from build123d import *

# Parameters (mm, degrees)
BOSS_EXTRUDE4_DEPTH = 5
SKETCH6_W           = 70
SKETCH6_H           = 70
BOSS_EXTRUDE5_DEPTH = 30
SKETCH8_R           = 3
CUT_EXTRUDE1_DEPTH  = 2
CUT_EXTRUDE2_START  = -30
CUT_EXTRUDE2_DEPTH  = 30
SKETCH10_W          = 140
SKETCH10_H          = 70
BOSS_EXTRUDE6_DEPTH = 2.5
FILLET1_R           = 10
CHAMFER1_SIZE       = 1.25
CHAMFER2_SIZE       = 1.25


with BuildPart() as part:
    # Sketch5 → Boss-Extrude4 (new body)
    with BuildSketch(Plane(origin=(0, 0, 0), x_dir=(1, 0, 0), z_dir=(0, 1, 0))):
        with BuildLine():
            Line((-22.5, -32.5), (22.5, -32.5))
            ThreePointArc((22.5, -32.5), (29.571067812, -29.571067812), (32.5, -22.5))
            Line((32.5, -22.5), (32.5, 22.5))
            ThreePointArc((32.5, 22.5), (29.571067812, 29.571067812), (22.5, 32.5))
            Line((22.5, 32.5), (-22.5, 32.5))
            ThreePointArc((-22.5, 32.5), (-29.571067812, 29.571067812), (-32.5, 22.5))
            Line((-32.5, 22.5), (-32.5, -22.5))
            ThreePointArc((-32.5, -22.5), (-29.571067812, -29.571067812), (-22.5, -32.5))
        make_face()
    extrude(amount=BOSS_EXTRUDE4_DEPTH)

    # Sketch6 → Boss-Extrude5 (add)
    with BuildSketch(Plane(origin=(0, 5, 0), x_dir=(1, 0, 0), z_dir=(0, 1, 0))):
        Rectangle(SKETCH6_W, SKETCH6_H)
    extrude(amount=BOSS_EXTRUDE5_DEPTH)

    # Sketch8 → Cut-Extrude1 (cut)
    with BuildSketch(Plane.XZ):
        with Locations(Location((26.037533906, -26.035533906, 0), (0, 0, 270))):
            Circle(SKETCH8_R)
        with Locations(Location((26.036533906, 26.036533906, 0), (0, 0, 270))):
            Circle(SKETCH8_R)
        with BuildLine():
            ThreePointArc((-23.035533906, 26.035533906), (-24.887483609, 28.807172503), (-28.156854249, 28.156854249))
            Line((-28.156854249, 28.156854249), (-23.914213562, 23.914213562))
            ThreePointArc((-23.914213562, 23.914213562), (-23.263895308, 24.887483609), (-23.035533906, 26.035533906))
        make_face()
        with BuildLine():
            Line((-23.914213562, 23.914213562), (-28.156854249, 28.156854249))
            ThreePointArc((-28.156854249, 28.156854249), (-28.156854249, 23.914213562), (-23.914213562, 23.914213562))
        make_face()
        with Locations(Location((-26.034533906, -26.036533906, 0), (0, 0, 270))):
            Circle(SKETCH8_R)
    extrude(amount=-CUT_EXTRUDE1_DEPTH, mode=Mode.SUBTRACT)

    # Mirror1: part across plane


with BuildPart() as part_1:
    add(part.part)
    add(part.part.mirror(Plane(origin=(-35, 35, -35), x_dir=(0, 0, 1), z_dir=(1, 0, 0))))

    # Sketch9 → Cut-Extrude2 (cut)
    with BuildSketch(Plane(origin=(0, 35, 0), x_dir=(1, 0, 0), z_dir=(0, 1, 0)).offset(CUT_EXTRUDE2_START)):
        with BuildLine():
            Line((22.5, 32.5), (-92.5, 32.5))
            ThreePointArc((-92.5, 32.5), (-99.571067812, 29.571067812), (-102.5, 22.5))
            Line((-102.5, 22.5), (-102.5, -22.5))
            ThreePointArc((-102.5, -22.5), (-99.571067812, -29.571067812), (-92.5, -32.5))
            Line((-92.5, -32.5), (22.5, -32.5))
            ThreePointArc((22.5, -32.5), (29.571067812, -29.571067812), (32.5, -22.5))
            Line((32.5, -22.5), (32.5, 22.5))
            ThreePointArc((32.5, 22.5), (29.571067812, 29.571067812), (22.5, 32.5))
        make_face()
    extrude(amount=CUT_EXTRUDE2_DEPTH, mode=Mode.SUBTRACT)


with BuildPart() as cut_extrude2_piece_1:
    # of the separate pieces the step leaves, piece 1, a body of its own (cut_extrude2_pieces)
    add(part_1.part.solids().sort_by_distance((35, 5, -35))[0])



with BuildPart() as cut_extrude2_piece_2:
    # of the separate pieces the step leaves, piece 2, a body of its own (cut_extrude2_pieces)
    add(part_1.part.solids().sort_by_distance((-22.5, 0, 32.5))[0])


with BuildPart() as cut_extrude2_piece_3:
    # of the separate pieces the step leaves, piece 3, a body of its own (cut_extrude2_pieces)
    add(part_1.part.solids().sort_by_distance((-92.5, 0, -32.5))[0])


with BuildPart() as cut_extrude2_piece_1_1:
    add(cut_extrude2_piece_1.part)

    add(cut_extrude2_piece_2.part)  # Boss-Extrude6 merges Cut-Extrude2 piece 2

    add(cut_extrude2_piece_3.part)  # Boss-Extrude6 merges Cut-Extrude2 piece 3
    # Sketch10 → Boss-Extrude6 (add)
    with BuildSketch(Plane.XZ.offset(-5)):
        with Locations((-35, 0)):
            Rectangle(SKETCH10_W, SKETCH10_H)
    extrude(amount=-BOSS_EXTRUDE6_DEPTH)

    # Fillet1
    fillet1_edges = [cut_extrude2_piece_1_1.edges().sort_by_distance(p)[0] for p in [
        (35, 20, 35),
        (35, 20, -35),
        (-105, 20, 35),
        (-105, 20, -35),
    ]]
    fillet(fillet1_edges, radius=FILLET1_R)

    # Chamfer1
    chamfer1_edges = [cut_extrude2_piece_1_1.edges().sort_by_distance(p)[0] for p in [
        (29.571067812, 7.5, -29.571067812),
        (-35, 7.5, -32.5),
        (-99.571067812, 7.5, -29.571067812),
        (-102.5, 7.5, 0),
        (-99.571067812, 7.5, 29.571067812),
        (-35, 7.5, 32.5),
        (29.571067812, 7.5, 29.571067812),
        (32.5, 7.5, 0),
    ]]
    chamfer(chamfer1_edges, length=CHAMFER1_SIZE)

    # Chamfer2
    chamfer2_edges = [cut_extrude2_piece_1_1.edges().sort_by_distance(p)[0] for p in [
        (-99.571067812, 35, 29.571067812),
        (-35, 35, 32.5),
        (29.571067812, 35, 29.571067812),
        (32.5, 35, 0),
        (29.571067812, 35, -29.571067812),
        (-35, 35, -32.5),
        (-99.571067812, 35, -29.571067812),
        (-102.5, 35, 0),
    ]]
    chamfer(chamfer2_edges, length=CHAMFER2_SIZE)


solid = cut_extrude2_piece_1_1.part
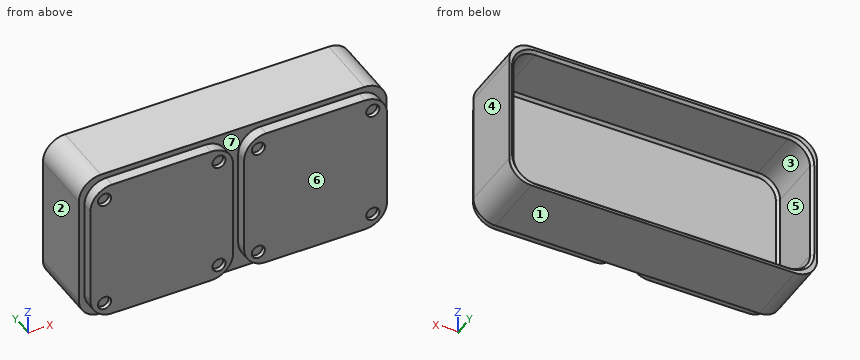
Verification items for the finished model (mm, model axes). Face numbers are marked on the shaded views. A direction names the side the tool comes from. Round coordinates to 2 decimals unless told otherwise and drop trailing zeros. Loops run counter-clockwise (first coordinate to the right, second up) from the corner with the lowest first, then second, coordinate; pieces in that order, holes last. Notation, with made-up numbers: (-6, -27) - (6, -27) arc R18 cw to (6, -2) - close; hole circle Ø8 at (76.25, 8.25). An arc over 180 degrees is marked (long way). Answer in a Markdown table with one row per item. Add a question column.
Q1. Gauge pin test, flat ends, axial feed: pin 1 (5.5 mm diameter, centred on x = -75, y = 3, fed in from +Z); pin 2 (10 mm diameter, centred on x = -65.5, z = 12, fed in from +Y); pin 3 (1.5 mm diameter, centred on y = 1.5, z = -11, fed in from +X); pin 4 (3 mm diameter, centred on x = -44, z = -26.5, fed in from -Y). Record the tip position at first contact, or that the pin passes through.
Q2. Section check A-A on x = -83. Enter the section's corners in (y, z).
Q3. Material ranges on line 1 (X direction, y = 17.5, z = 1.5); line 2 (Z direction, x = 15.5, y = 27.5); line 3 (Y direction, x = 20, z = 22), recorded low to high.
Q4. Tool access check on the marked faces 5, 6 and 7. Record the directions out of +Z, -Z, +X, -X, +Y, -Y that give a thin tool (end or side, any length) a straight path to the whole face; none if there is none.
Q5. Section check C-C on z = -2. Enter the section's corners in (x, y), plus the area to 3 significant figures.
Q6. Release check for a two-part mould opening along X. For the marked faces 1, 2, 3 and 4 record: pulls with the +X half, pulls with the -X half, needs draft (parallel to the pull), parting line crosses it, or undercut.
Q7. Section check B-B on y = 12. Enter the section's corners in (x, z), plus the area to 4 significant figures.
Found:
| question | item | result |
|---|---|---|
| 1 | pin 1 | stops at z = 35 |
| 1 | pin 2 | stops at y = 7.5 |
| 1 | pin 3 | stops at x = 32.5 |
| 1 | pin 4 | stops at y = 2 |
| 2 | outline | (0, -32.5) - (5, -32.5) - (5, -35) - (35, -35) - (35, -33.75) - (33.75, -32.5) - (8.75, -32.5) - (7.5, -31.25) - (7.5, 31.25) - (8.75, 32.5) - (33.75, 32.5) - (35, 33.75) - (35, 35) - (5, 35) - (5, 32.5) - (0, 32.5) - close |
| 3 | line 1 | x = -105 to -102.5, 32.5 to 35 |
| 3 | line 2 | z = -35 to -32.5, 32.5 to 35 |
| 3 | line 3 | y = 0 to 7.5 |
| 4 | face 5 | +Y |
| 4 | face 6 | +Z, -Z, +X, -X, -Y |
| 4 | face 7 | -Y |
| 5 | outline | (-105, 5) - (-102.5, 5) - (-102.5, 0) - (-37.5, 0) - (-37.5, 5) - (-32.5, 5) - (-32.5, 0) - (32.5, 0) - (32.5, 5) - (35, 5) - (35, 35) - (33.75, 35) - (32.5, 33.75) - (32.5, 8.75) - (31.25, 7.5) - (-101.25, 7.5) - (-102.5, 8.75) - (-102.5, 33.75) - (-103.75, 35) - (-105, 35) - close |
| 5 | area | 1,140 mm² |
| 6 | face 1 | needs draft |
| 6 | face 2 | pulls with the -X half |
| 6 | face 3 | undercut |
| 6 | face 4 | pulls with the +X half |
| 7 | outline | (-105, -25) arc R10 ccw to (-95, -35) - (25, -35) arc R10 ccw to (35, -25) - (35, 25) arc R10 ccw to (25, 35) - (-95, 35) arc R10 ccw to (-105, 25) - close; hole (-102.5, -22.5) arc R10 ccw to (-92.5, -32.5) - (22.5, -32.5) arc R10 ccw to (32.5, -22.5) - (32.5, 22.5) arc R10 ccw to (22.5, 32.5) - (-92.5, 32.5) arc R10 ccw to (-102.5, 22.5) - close |
| 7 | area | 1,025 mm² |
